CAD build for the part. Positions are in the model's coordinates, mm. A direction names the side the tool comes from. Give positions to 0.01 mm unless a question says otherwise; leave off trailing zeros. Write each loop counter-clockwise with the first axis right and the second up, starting at its lowest first coordinate (ties: lowest second). Pieces come first, ordered by that corner, then holes. Notation, with made-up numbers: (43.25, 26.25) - (55.25, 26.25) arc R28 ccw to (55.25, 60.25) - close; hole circle Ø8 at (10.25, 61). An arc over 180 degrees is marked (long way). Put each result on its own line as item: value. Start each with the question number.
1. Wall check: line 1 (Y direction, x = -14.5, z = 1.85); line 2 (X direction, y = -0.5, z = 4); line 3 (X direction, y = -1, z = 3.55). Give the ranges that are in metal, low to high.
2. Cut at D-D on z = 1.35. List the corners of the cut face in (x, y) (3 decimals).
3. Cut at C-C on y = 30. List the corners of the cut face in (x, z).
4. Cut at A-A on y = -13.5. List the corners of the cut face in (x, z), and give its area (3 significant figures).
5. Cut at B-B on x = 9.5. List the corners of the cut face in (y, z), and give its area (3 significant figures).
6. Tool access for faces 1 (the flat face through (9, 1, 5)), 2 (the cylindrical face through (5.25, 29.88, 2.54)): list every direction of +Z, -Z, +X, -X, +Y, -Y with a clear straight run to the whole face (end or side of a thin tool).
7. Drop flat-ended pins along their axis: pin 1 (1 mm diameter, centred on y = -31.5, z = 2.5, fed in from -X); pin 2 (1.5 mm diameter, centred on y = -24.5, z = 2, fed in from -X). Give the stop position or say it passes through.
8. Mould opens along X. For faces 3 (the cylindrical face through (24.98, 8.82, 2.54)), 4 (the flat face through (9, 1, 0)), 5 (the cylindrical face through (20.765, -39.923, 2.465)) say: +X half, -X half, draft (parallel to the pull), parting line (faces both ways), or undercut.
from build123d import *

# Parameters (mm, degrees)
CROQUIS1_R            = 45
DISCO_DEPTH           = 5
CORTAR_EXTRUIR6_DEPTH = 5


with BuildPart() as part:
    # Croquis1 → Disco (new body)
    with BuildSketch(Plane.XY):
        Circle(CROQUIS1_R)
    extrude(amount=DISCO_DEPTH)

    # Croquis6 → Cortar-Extruir6 (cut)
    with BuildSketch(Plane.XY.offset(5)):
        with BuildLine():
            ThreePointArc((-30.527395483, -17.625), (-4.464035413, -25.86746934), (6.062177826, -0.639788633))
            ThreePointArc((6.062177826, -0.639788633), (18.906715666, 0.249805468), (21.434128744, -12.375))
            ThreePointArc((21.434128744, -12.375), (23.355762114, -19.54663337), (30.527395483, -17.625))
            ThreePointArc((30.527395483, -17.625), (24.633903286, 9.067766599), (-2.477015704, 5.569894316))
            ThreePointArc((-2.477015704, 5.569894316), (-9.669695714, 16.248793335), (0, 24.75))
            ThreePointArc((0, 24.75), (5.25, 30), (0, 35.25))
            ThreePointArc((0, 35.25), (-20.169867874, 16.799702741), (-3.585162122, -4.930105684))
            ThreePointArc((-3.585162122, -4.930105684), (-9.237019952, -16.498598803), (-21.434128744, -12.375))
            ThreePointArc((-21.434128744, -12.375), (-28.605762114, -10.45336663), (-30.527395483, -17.625))
        make_face()
    extrude(amount=-CORTAR_EXTRUIR6_DEPTH, mode=Mode.SUBTRACT)


solid = part.part
Report:
1. line 1: y = -42.6 to -27.69, -17.13 to 0.86, 29.14 to 42.6
1. line 2: x = -45 to -13.03, 6.2 to 19.78, 31.99 to 45
1. line 3: x = -44.99 to -12.41, 6.19 to 20.26, 32.17 to 44.99
2. outline: circle Ø90 at (0, 0); hole (-30.527, -17.625) arc R20.25 ccw to (6.062, -0.64) arc R9.75 cw to (21.434, -12.375) arc R5.25 ccw to (30.527, -17.625) arc R20.25 ccw to (-2.477, 5.57) arc R9.75 cw to (0, 24.75) arc R5.25 ccw to (0, 35.25) arc R20.25 ccw to (-3.585, -4.93) arc R9.75 cw to (-21.434, -12.375) arc R5.25 ccw to start
3. outline: (-33.54, 0) - (-13.6, 0) - (-13.6, 5) - (-33.54, 5) - close; (5.25, 0) - (33.54, 0) - (33.54, 5) - (5.25, 5) - close
4. outline: (-42.93, 0) - (-31.01, 0) - (-31.01, 5) - (-42.93, 5) - close; (-20.68, 0) - (-5.31, 0) - (-5.31, 5) - (-20.68, 5) - close; (6.35, 0) - (20.95, 0) - (20.95, 5) - (6.35, 5) - close; (32.33, 0) - (42.93, 0) - (42.93, 5) - (32.33, 5) - close
4. area: 262 mm²
5. outline: (-43.99, 0) - (1.6, 0) - (1.6, 5) - (-43.99, 5) - close; (12.45, 0) - (43.99, 0) - (43.99, 5) - (12.45, 5) - close
5. area: 386 mm²
6. face 1: +Z, +X, -X, +Y, -Y
6. face 2: +Z, -Z
7. pin 1: stops at x = -32.62
7. pin 2: stops at x = -38.22
8. face 3: undercut
8. face 4: draft
8. face 5: parting line
